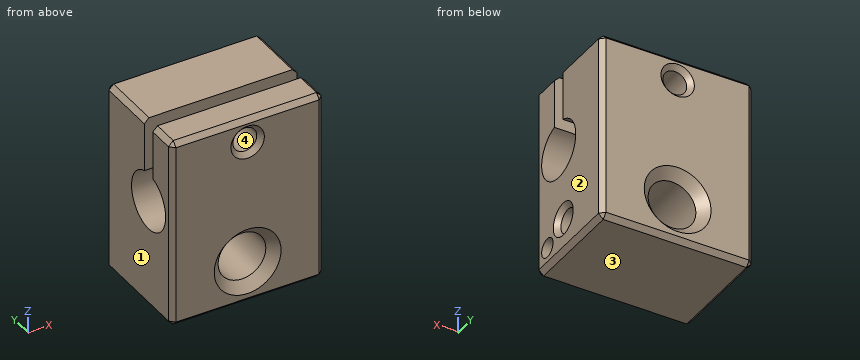
```python
from build123d import *

# Parameters (mm, degrees)
SKETCH_1_W            = 20
SKETCH_1_H            = 11.5
EXTRUDE_1_DEPTH       = 8
CUT_EXTRUDE_1_REACH   = 18
HOLE_WIZARD_M31_D     = 2.5
HOLE_WIZARD_M31_DEPTH = 11.5
HOLE_WIZARD_M31_TIP   = 0.751075774
HOLE_WIZARD_M61_D     = 5
HOLE_WIZARD_M61_DEPTH = 11.5
CHAMFER_1_SIZE        = 0.5
CHAMFER_2_SIZE        = 1
HOLE_WIZARD_M32_D     = 2.5
HOLE_WIZARD_M32_DEPTH = 3.8
HOLE_WIZARD_M32_TIP   = 0.751075774
CHAMFER_3_SIZE        = 0.5
HOLE_WIZARD_1_D       = 1.5
HOLE_WIZARD_1_DEPTH   = 4.4
HOLE_WIZARD_1_TIP     = 0.450645464
HOLE_WIZARD_2_D       = 2
HOLE_WIZARD_2_DEPTH   = 2
HOLE_WIZARD_2_TIP     = 0.600860619
CHAMFER_4_SIZE        = 0.5


with BuildPart() as part:
    # Эскиз1 → Бобышка-Вытянуть1 (new body, symmetric)
    with BuildSketch(Plane(origin=(0, 0, 0), x_dir=(0, 0, -1), z_dir=(1, 0, 0))):
        Rectangle(SKETCH_1_W, SKETCH_1_H)
    extrude(amount=EXTRUDE_1_DEPTH, both=True)

    # Эскиз2 → Вырез-Вытянуть1 (cut, up to next)
    with BuildSketch(Plane(origin=(8, 0, 0), x_dir=(0, 0, -1), z_dir=(1, 0, 0)), mode=Mode.PRIVATE) as cut_extrude_1_sk1:
        with BuildLine():
            Line((-10, -1), (-4.40473751, -1))
            ThreePointArc((-4.40473751, -1), (1.5, -1.75), (-4.40473751, -2.5))
            Line((-4.40473751, -2.5), (-10, -2.5))
            Line((-10, -2.5), (-10, -1))
        make_face()
    cut_extrude_1_tool1 = extrude(cut_extrude_1_sk1.sketch, amount=-CUT_EXTRUDE_1_REACH, mode=Mode.PRIVATE) & part.part
    add(cut_extrude_1_tool1.solids().sort_by_distance((8, -1.75, 2.800956))[0], mode=Mode.SUBTRACT)

    # Отверстие обработанное метчиком M31
    with Locations(Plane(origin=(0, 5.75, 0), x_dir=(-1, 0, 0), z_dir=(0, 1, 0))):
        with Locations((0, 7.5)):
            Hole(HOLE_WIZARD_M31_D / 2, depth=HOLE_WIZARD_M31_DEPTH)
            with Locations((0, 0, -(HOLE_WIZARD_M31_DEPTH + HOLE_WIZARD_M31_TIP / 2))):  # 118° drill point
                Cone(0, HOLE_WIZARD_M31_D / 2, HOLE_WIZARD_M31_TIP, mode=Mode.SUBTRACT)

    # Отверстие обработанное метчиком M61
    with Locations(Plane(origin=(0, 5.75, 0), x_dir=(-1, 0, 0), z_dir=(0, 1, 0))):
        with Locations((0, -5.5)):
            Hole(HOLE_WIZARD_M61_D / 2, depth=HOLE_WIZARD_M61_DEPTH)

    # Фаска1
    chamfer_1_edges = [part.edges().sort_by_distance(p)[0] for p in [
        (-1.25, 5.75, 7.5),
        (-1.25, -5.75, 7.5),
    ]]
    chamfer(chamfer_1_edges, length=CHAMFER_1_SIZE)

    # Фаска2
    chamfer_2_edges = [part.edges().sort_by_distance(p)[0] for p in [
        (-2.5, 5.75, -5.5),
        (-2.5, -5.75, -5.5),
    ]]
    chamfer(chamfer_2_edges, length=CHAMFER_2_SIZE)

    # Отверстие обработанное метчиком M32
    with Locations(Plane(origin=(8, 0, 0), x_dir=(0, 0, -1), z_dir=(1, 0, 0))):
        with Locations((6.5, -0.95)):
            Hole(HOLE_WIZARD_M32_D / 2, depth=HOLE_WIZARD_M32_DEPTH)
            with Locations((0, 0, -(HOLE_WIZARD_M32_DEPTH + HOLE_WIZARD_M32_TIP / 2))):  # 118° drill point
                Cone(0, HOLE_WIZARD_M32_D / 2, HOLE_WIZARD_M32_TIP, mode=Mode.SUBTRACT)

    # Фаска3
    chamfer_3_edges = [part.edges().sort_by_distance(p)[0] for p in [
        (8, -0.95, -7.75),
    ]]
    chamfer(chamfer_3_edges, length=CHAMFER_3_SIZE)

    # Отверстие1
    with Locations(Plane(origin=(8, 0, 0), x_dir=(0, 0, -1), z_dir=(1, 0, 0))):
        with Locations((8, -3.75)):
            Hole(HOLE_WIZARD_1_D / 2, depth=HOLE_WIZARD_1_DEPTH)
            with Locations((0, 0, -(HOLE_WIZARD_1_DEPTH + HOLE_WIZARD_1_TIP / 2))):  # 118° drill point
                Cone(0, HOLE_WIZARD_1_D / 2, HOLE_WIZARD_1_TIP, mode=Mode.SUBTRACT)

    # Отверстие2
    with Locations(Plane(origin=(8, 0, 0), x_dir=(0, 0, -1), z_dir=(1, 0, 0))):
        with Locations((8, -3.75)):
            Hole(HOLE_WIZARD_2_D / 2, depth=HOLE_WIZARD_2_DEPTH)
            with Locations((0, 0, -(HOLE_WIZARD_2_DEPTH + HOLE_WIZARD_2_TIP / 2))):  # 118° drill point
                Cone(0, HOLE_WIZARD_2_D / 2, HOLE_WIZARD_2_TIP, mode=Mode.SUBTRACT)

    # Фаска4
    chamfer_4_edges = [part.edges().sort_by_distance(p)[0] for p in [
        (8, 0, -10),
        (8, 5.75, 0),
        (-8, -4.125, 10),
        (8, -4.125, 10),
        (8, 2.375, 10),
        (-8, 5.75, 0),
        (-8, 0, -10),
        (-8, -5.75, 0),
        (-8, 2.375, 10),
        (8, -5.75, 0),
        (0, 5.75, 10),
        (0, 5.75, -10),
        (0, -5.75, -10),
        (0, -5.75, 10),
    ]]
    chamfer(chamfer_4_edges, length=CHAMFER_4_SIZE)


solid = part.part
```
Part model, mm, in its own coordinate system. Face numbers are marked on the shaded views. Coordinates: 2 decimals unless noted, no trailing zeros. Order: outer loops, then holes, each group sorted by start corner. A loop starts at its lowest first (then second) coordinate and runs counter-clockwise, first axis right, second up. Notation, with made-up numbers: (37, 84) -> (71, 84) arc R12 ccw to (71, 89) -> close; hole circle Ø3 at (83, 81). An arc over 180 degrees is marked (long way). Put each result on its own line as item: value. Start each with the question number.
(1) Band-saw the part on A-A (x = 0). Count the separate pieces of the cut face and the enclosed holes in it, then the cut area to 3 significant figures.
(2) Band-saw the part on B-B (y = 3.25). Give the cut face in (x, z), then the cut area to 3 significant figures.
(3) Pin check, flat tips, straight feed: pin 1 Ø3 at (x, z) = (0, 7.5) entering from -Y; pin 2 Ø2 at (y, z) = (-0.95, -6.5) entering from +X. Stop position of each tip, or through.
(4) Mould opens along X. For the marked faces 1, 2, 3 and 4 say: pulls with the +X half, pulls with the -X half, needs draft (parallel to the pull), parting line crosses it, or undercut.
(5) Probe line 1 along Y through (x, z) = (-4.25, 7.75); line 2 along Z through (x, y) = (7.55, -3.75); line 3 along Z through (x, y) = (7.1, -3.75). List the from-to ranges inside material, lowest first. Write a range as [from, to].
(6) Band-saw the part on D-D (z = 7.5). Give the cut face in (x, y), then the cut area to 3 significant figures.
(7) Band-saw the part on C-C (z = 1.5). Give the cut face in (x, y), then the cut area to 3 significant figures.
Determined:
1. separate pieces: 4
1. enclosed holes: 0
1. area: 108 mm²
2. outline: (-8, -9.5) -> (-7.5, -10) -> (7.5, -10) -> (8, -9.5) -> (8, 9.5) -> (7.5, 10) -> (-7.5, 10) -> (-8, 9.5) -> close; hole circle Ø5 at (0, -5.5); hole circle Ø2.5 at (0, 7.5)
2. area: 295 mm²
3. pin 1: stops at y = -5.5
3. pin 2: stops at x = 4.05
4. face 1: pulls with the -X half
4. face 2: pulls with the +X half
4. face 3: needs draft
4. face 4: undercut
5. line 1: y = [-5.75, -2.5], [-1, 5.75]
5. line 2: z = [-9.95, -9], [-7, -0.74], [3.74, 9.95]
5. line 3: z = [-10, -9], [-7, -0.74], [3.74, 10]
6. outline: (-8, -5.25) -> (-7.5, -5.75) -> (-1.75, -5.75) -> (-1.25, -5.25) -> (-1.25, -2.5) -> (-8, -2.5) -> close; (-8, -1) -> (-1.25, -1) -> (-1.25, 5.25) -> (-1.75, 5.75) -> (-7.5, 5.75) -> (-8, 5.25) -> close; (1.25, -5.25) -> (1.75, -5.75) -> (7.5, -5.75) -> (8, -5.25) -> (8, -2.5) -> (1.25, -2.5) -> close; (1.25, -1) -> (8, -1) -> (8, 5.25) -> (7.5, 5.75) -> (1.75, 5.75) -> (1.25, 5.25) -> close
6. area: 134 mm²
7. outline: (-8, -5.25) -> (-7.5, -5.75) -> (7.5, -5.75) -> (8, -5.25) -> (8, -4.75) -> (-8, -4.75) -> close; (-8, 1.25) -> (8, 1.25) -> (8, 5.25) -> (7.5, 5.75) -> (-7.5, 5.75) -> (-8, 5.25) -> close
7. area: 87.5 mm²
